Design review of the part built by this model. Coordinates are the model's own, in mm. Give positions to 0.01 mm unless a question says otherwise; leave off trailing zeros. Order: outer loops, then holes, each group sorted by start corner. A loop starts at its lowest first (then second) coordinate and runs counter-clockwise, first axis right, second up. Notation, with made-up numbers: (-11.75, 80) -> (0.25, 80) arc R21 cw to (0.25, 115) -> close; hole circle Ø1 at (14, 47.5). An arc over 180 degrees is marked (long way). Answer in a Markdown table with one row per item. Add a question column.
```python
from build123d import *

# Parameters (mm, degrees)
SKETCH_1_R               = 15
SKETCH_1_R_2             = 4.05
EXTRUDE_1_DEPTH          = 10
CUT_EXTRUDE_1_DEPTH      = 24.452078799
CUT_EXTRUDE_1_DEPTH_BACK = 24.452078799
SKETCH_2_R               = 1.3
SKETCH_3_R               = 1.65
SKETCH_3_R_2             = 1.3
CUT_EXTRUDE_2_DEPTH      = 24.452078982


with BuildPart() as part:
    # ｽｹｯﾁ1 → ﾎﾞｽ - 押し出し1 (new body)
    with BuildSketch(Plane(origin=(0, 0, 0), x_dir=(0, 0, -1), z_dir=(1, 0, 0))):
        Circle(SKETCH_1_R)
        Circle(SKETCH_1_R_2, mode=Mode.SUBTRACT)
    extrude(amount=EXTRUDE_1_DEPTH)

    # ｽｹｯﾁ2 → ｶｯﾄ - 押し出し1 (cut, two sides: drawn at the far end of the back side and taken through both)
    with BuildSketch(Plane(origin=(0, 0, 0), x_dir=(1, 0, 0), z_dir=(0, 1, 0)).offset(-CUT_EXTRUDE_1_DEPTH_BACK)):
        with Locations(Location((5, 0, 0), (0, 0, 270))):
            Circle(SKETCH_2_R)
    extrude(amount=CUT_EXTRUDE_1_DEPTH + CUT_EXTRUDE_1_DEPTH_BACK, mode=Mode.SUBTRACT)

    # ｽｹｯﾁ3 → ｶｯﾄ - 押し出し2 (cut, through all)
    with BuildSketch(Plane(origin=(10, 0, 0), x_dir=(0, 0, -1), z_dir=(1, 0, 0))):
        with Locations((0, 10)):
            Circle(SKETCH_3_R)
        with Locations(Location((0, -10, 0), (0, 0, 180))):
            Circle(SKETCH_3_R)
        with Locations((-5.5, 9.526279442)):
            Circle(SKETCH_3_R_2)
        with Locations(Location((5.5, -9.526279442, 0), (0, 0, 180))):
            Circle(SKETCH_3_R_2)
    extrude(amount=-CUT_EXTRUDE_2_DEPTH, mode=Mode.SUBTRACT)


solid = part.part
```
1) Add section C-C, the plane x = 5. Write out the cut boundary in (y, z).
2) Add section D-D, the plane z = -5.5. Write out the cut boundary in (x, y), and give its area (3 significant figures).
3) For L1, parallel to Y at x = 8.25, z = 0; L2, parallel to X at y = -12.55, z = 0; L3, parallel to Z at x = 5.25, y = -8.5, list the stretches that pass through material, from the lowest coordinate up.
4) Clearance check with flat-ended pins moving along their axes: P1, Ø1.5, axis at x = 6, y = 7, coming from the +Z side; P2, Ø1.5, axis at x = 5, y = 2, coming from the +Z side; P3, Ø3, axis at x = 2.5, z = 12, coming from the +Y side. State where each tip first meets the part, or that it passes through.
5) Add section B-B, the plane y = 0. Write out the cut boundary in (x, z).
6) Mouldability with a two-part tool opening along X and no side actions: class faces 1 (the face through (4.5, -6.4, 1.2)), 2 (the face through (0, -3, -3)), 3 (the face through (10, -3, -3)), 4 (the face through (5.07, 8.373, 4.9)) as +X half, -X half, draft (parallel to the pull), parting line (faces both ways), or undercut.
7) Add section A-A, the plane z = 0. Give the number of separate pieces and of enclosed holes in the cut face, and give its area (3 significant figures).
Verdict:
| question | item | result |
|---|---|---|
| 1 | outline | (-14.94, -1.3) arc R15 ccw to (14.94, -1.3) -> (11.02, -1.3) arc R1.65 cw to (8.98, -1.3) -> (3.84, -1.3) arc R4.05 cw to (-3.84, -1.3) -> (-8.98, -1.3) arc R1.65 cw to (-11.02, -1.3) -> close; (-14.94, 1.3) -> (-11.02, 1.3) arc R1.65 cw to (-8.98, 1.3) -> (-3.84, 1.3) arc R4.05 cw to (3.84, 1.3) -> (8.98, 1.3) arc R1.65 cw to (11.02, 1.3) -> (14.94, 1.3) arc R15 ccw to start; hole circle Ø2.6 at (-9.53, -5.5); hole circle Ø2.6 at (9.53, 5.5) |
| 2 | outline | (0, -13.96) -> (10, -13.96) -> (10, -10.83) -> (0, -10.83) -> close; (0, -8.23) -> (10, -8.23) -> (10, 13.96) -> (0, 13.96) -> close |
| 2 | area | 253 mm2 |
| 3 | L1 | y = -15 to -11.65, -8.35 to -4.05, 4.05 to 8.35, 11.65 to 15 |
| 3 | L2 | x = 0 to 3.7, 6.3 to 10 |
| 3 | L3 | z = -12.36 to -6.3, -4.7 to -1.28, 1.28 to 12.36 |
| 4 | P1 | stops at z = 13.64 |
| 4 | P2 | stops at z = 14.95 |
| 4 | P3 | stops at y = 10.71 |
| 5 | outline | (0, -15) -> (10, -15) -> (10, -4.05) -> (0, -4.05) -> close; (0, 4.05) -> (10, 4.05) -> (10, 15) -> (0, 15) -> close |
| 6 | face 1 | undercut |
| 6 | face 2 | -X half |
| 6 | face 3 | +X half |
| 6 | face 4 | draft |
| 7 | separate pieces | 8 |
| 7 | enclosed holes | 0 |
| 7 | area | 113 mm2 |
